```python
from build123d import *

# Parameters (mm, degrees)
F0_W     = 501.65
F0_H     = 74.422
F0_H_2   = 74.676
F1_DEPTH = 66.675
F2_DEPTH = 387.35
F3_R     = 1.5875


with BuildPart() as f1:
    # F0 (on Front) → F1 (new body)
    with BuildSketch(Plane.XZ):
        with Locations((-66.268259, 59.105321)):
            Rectangle(F0_W, F0_H)
        Polygon((-317.093259, 21.894321), (-501.243259, 21.894321), (-501.243259, -333.705679), (-317.093259, -333.705679), (184.556741, -333.705679), (184.556741, 21.894321), align=None)
        with Locations((-66.268259, -371.043679)):
            Rectangle(F0_W, F0_H_2)
    extrude(amount=F1_DEPTH)

    # F0 (on Front) → F2 (join)
    with BuildSketch(Plane.XZ):
        Polygon((-317.093259, 21.894321), (-501.243259, 21.894321), (-501.243259, -333.705679), (-317.093259, -333.705679), (184.556741, -333.705679), (184.556741, 21.894321), align=None)
    extrude(amount=F2_DEPTH)

    # F3
    f3_edges = [f1.edges().sort_by_distance(p)[0] for p in [
        (-158.343259, -387.35, 21.894321),
        (-501.243259, -193.675, 21.894321),
        (184.556741, -227.0125, 21.894321),
        (184.556741, -387.35, -155.905679),
        (184.556741, -227.0125, -333.705679),
        (-158.343259, -387.35, -333.705679),
        (-501.243259, -387.35, -155.905679),
        (-501.243259, -193.675, -333.705679),
    ]]
    fillet(f3_edges, radius=F3_R)


solid = f1.part
```
For this review, take the finished solid that the model builds, in its own axes (mm). A direction names the side the tool comes from. Round coordinates to 2 decimals unless told otherwise and drop trailing zeros. Write each loop counter-clockwise with the first axis right and the second up, starting at its lowest first coordinate (ties: lowest second). Pieces come first, ordered by that corner, then holes. Notation, with made-up numbers: (72, 43.5) - (78, 43.5) arc R31 ccw to (78, 75.5) - close; hole circle Ø1 at (22.25, -29). An arc over 180 degrees is marked (long way). Answer as a JSON object with one key per item and string values.
1. We need section A-A on y = -49. Give the boundary of the cut face in (x, z) (1 decimal), then the cut area to 3 significant figures.
Response values:
{"outline": "(-501.2, -332.1) arc R1.6 ccw to (-499.7, -333.7) - (-317.1, -333.7) - (-317.1, -408.4) - (184.6, -408.4) - (184.6, 96.3) - (-317.1, 96.3) - (-317.1, 21.9) - (-499.7, 21.9) arc R1.6 ccw to (-501.2, 20.3) - close", "area": "319,000 mm2"}
2. Tool access review of faces 1 (the face through (-317.093, -33, 59)), 2 (the face through (-70, -66.675, 59)), 3 (the face through (-163, 0, -152)), 4 (the face through (-317.093, -33, -372)), 5 (the face through (-70, -66.675, -370)): name each direction out of +Z, -Z, +X, -X, +Y, -Y from which nothing blocks a thin tool from reaching the whole face with its end or side.
Response values:
{"face 1": "+Z, -X, +Y, -Y", "face 2": "+Z, +X, -X, -Y", "face 3": "+Z, -Z, +X, -X, +Y", "face 4": "-Z, -X, +Y, -Y", "face 5": "-Z, +X, -X, -Y"}
3. We need section D-D on y = -98.5. Give the boundary of the cut face in (x, z) (1 decimal), then the cut area to 3 significant figures.
Response values:
{"outline": "(-501.2, -332.1) arc R1.6 ccw to (-499.7, -333.7) - (183, -333.7) arc R1.6 ccw to (184.6, -332.1) - (184.6, 20.3) arc R1.6 ccw to (183, 21.9) - (-499.7, 21.9) arc R1.6 ccw to (-501.2, 20.3) - close", "area": "244,000 mm2"}
4. To check wall thickness, follow line 1 along Z through (x, y) = (14, -368); line 2 along Y through (x, z) = (145, -379.5) (3 decimals); line 3 along X through (y, z) = (-38.5, -358). State the ranges of each line that lie inside material, in increasing order.
Response values:
{"line 1": "z = -333.71 to 21.89", "line 2": "y = -66.675 to 0", "line 3": "x = -317.09 to 184.56"}
5. For pin 1 Ø12 at (x, z) = (40, -349.5) entering from +Y; pin 2 Ø6 at (x, y) = (-3.5, -164) entering from +Z; pin 3 Ø23 at (x, z) = (-140.5, -379) entering from -Y (3 decimals), all flat-tipped, find the tip position at first contact; note any pin that passes through.
Response values:
{"pin 1": "stops at y = 0", "pin 2": "stops at z = 21.89", "pin 3": "stops at y = -66.675"}
